Geometry: see drawing. Coordinates: mm, zero at the bounding-box minimum. Round coordinates to 2 decimals unless told otherwise and drop trailing zeros. Write each loop counter-clockwise with the first axis right and the second up, starting at its lowest first coordinate (ties: lowest second). Pieces come first, ordered by that corner, then holes. Notation, with made-up numbers: M 82,-4.75 L 115,-4.75 A32 ccw 115,32.25 Z; hole C 42.25,-39 d2. An arc over 180 degrees is marked long. Use one line per item in the form item = value. Start each with the question number.
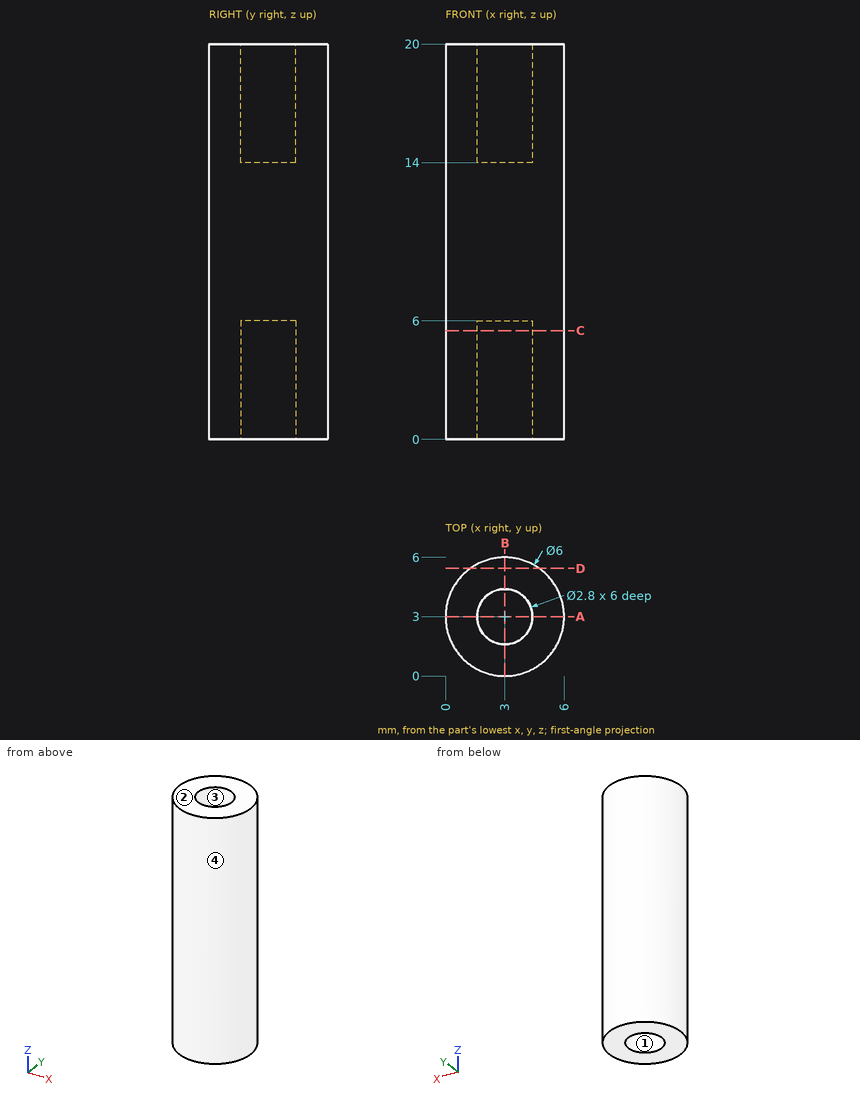
Item 1: Cut plane A-A (y = 3). Output: boundary loops of the cut face in (x, z), plus the area to 3 significant figures.
Item 2: Ray query, line 1 (Y direction, x = 3, z = 16.8); line 2 (Z direction, x = 2.85, y = 2.75); line 3 (X direction, y = 3.1, z = 7.75). Return the intervals inside material, ascending. Write a range as from..to.
Item 3: Draft query along Y for the marked faces 1, 2, 3 and 4. Return one class per face: +Y half, -Y half, draft (parallel to the pull), parting line (faces both ways), or undercut.
Item 4: First-contact query: pin 1 (2 mm diameter, centred on x = 4.5, z = 16.5, fed in from +Y). Flat tip, straight axial feed; report the tip coordinate or a pass-through.
Item 5: Cut plane D-D (y = 5.45). Output: boundary loops of the cut face in (x, z).
Item 6: Cut plane C-C (z = 5.5). Output: boundary loops of the cut face in (x, y).
Final values:
q1.outline = M 0,0 L 1.6,0 L 1.6,6 L 4.4,6 L 4.4,0 L 6,0 L 6,20 L 4.4,20 L 4.4,14 L 1.6,14 L 1.6,20 L 0,20 Z
q1.area = 86.4 mm^2
q2.line_1 = 0..1.6, 4.4..6
q2.line_2 = 6..14
q2.line_3 = 0..6
q3.face_1 = undercut
q3.face_2 = draft
q3.face_3 = undercut
q3.face_4 = parting line
q4.pin_1 = 5.96
q5.outline = M 1.27,0 L 4.73,0 L 4.73,20 L 1.27,20 Z
q6.outline = C 3,3 d6; hole C 3,3 d2.8
